Here's how the part is built. I have some questions about the finished solid (model axes, mm). Face numbers are marked on the shaded views. A direction names the side the tool comes from. Give positions to 0.01 mm unless a question says otherwise; leave off trailing zeros. Write each loop counter-clockwise with the first axis right and the second up, starting at its lowest first coordinate (ties: lowest second). Pieces come first, ordered by that corner, then holes. Notation, with made-up numbers: (-35, 73.5) - (-27, 73.5) arc R25 ccw to (-27, 96.5) - close; hole circle Ø11 at (50, -6). An arc over 180 degrees is marked (long way). Use a Markdown table: item, result.
Autodesk Inventor part; units mm, degrees
ref_plane "YZ Plane" through (0, 0, 0) normal (1, 0, 0) x (0, 1, 0)
ref_plane "XZ Plane" through (0, 0, 0) normal (0, 1, 0) x (-1, 0, 0)
ref_plane "XY Plane" through (0, 0, 0) normal (0, 0, 1) x (1, 0, 0)
sketch "Sketch1" plane through (0, 0, 0) normal (0, 1, 0) x (-1, 0, 0)
  line L0 (-11.9316, 12.465) -> (11.9317, 12.465)
  line L1 (11.9317, 12.465) -> (11.9316, -12.465)
  line L2 (11.9316, -12.465) -> (-11.9317, -12.465)
  line L3 (-11.9317, -12.465) -> (-11.9316, 12.465)
  line L4 (-11.9316, 12.465) -> (11.9316, -12.465) construction
  line L5 (11.9317, 12.465) -> (-11.9317, -12.465) construction
  circle A0 centre (10.0076, 9.4933) radius 1.0351
  line L6 (0, 0) -> (10.0076, 0) construction
  line L7 (10.0076, 0) -> (10.0076, 9.4933) construction
  line L8 (4.7752, 0) -> (4.7752, 3.1605) construction
  circle A1 centre (10.0076, -9.4933) radius 1.0351
  circle A2 centre (-0.4572, 9.4933) radius 1.0351
  circle A3 centre (-0.4572, -9.4933) radius 1.0351
  dimension "d0" = 24.9301
  dimension "d1" = 23.8633
  dimension "d2" = 2.0701
  dimension "d3" = 1.9241
  dimension "d5" = 5.2324
  dimension "d16" = 18.9865
extrude "Extrusion1" add sketch "Sketch1" along normal blind 1.016
sketch "Sketch2" plane through (0, 1.016, 0) normal (0, 1, 0) x (1, 0, 0)
  line L0 (4.2101, -4.21) -> (-4.21, -4.21)
  line L1 (-4.21, -4.21) -> (-4.21, 4.21)
  line L2 (-4.21, 4.21) -> (4.2101, 4.2101)
  line L3 (4.2101, 4.2101) -> (4.2101, -4.21)
  line L4 (4.2101, -4.21) -> (-4.21, 4.21) construction
  line L5 (-4.21, -4.21) -> (4.2101, 4.2101) construction
  point P0 (0, 0)
  dimension "d8" = 8.4201
  dimension "d9" = 8.4201
extrude "Extrusion2" add sketch "Sketch2" along normal blind 3.81
sketch "Sketch3" plane through (0, 0, 0) normal (0, -1, 0) x (1, 0, 0)
  line L0 (11.9316, 12.465) -> (11.9317, -12.465)
  line L1 (6.5977, 9.7536) -> (11.9317, 9.7536)
  line L2 (11.9317, 9.7536) -> (11.9317, -9.7536)
  line L3 (11.9317, -9.7536) -> (6.5977, -9.7536)
  line L4 (6.5977, -9.7536) -> (6.5977, 9.7536)
  line L5 (6.5977, 9.7536) -> (11.9317, -9.7536) construction
  line L6 (11.9317, 9.7536) -> (6.5977, -9.7536) construction
  line L7 (0, 0) -> (9.2647, 0) construction
  dimension "d12" = 5.334
  dimension "d13" = 19.5072
extrude "Extrusion3" add sketch "Sketch3" along normal blind 2.1844
properties part number "Camera"
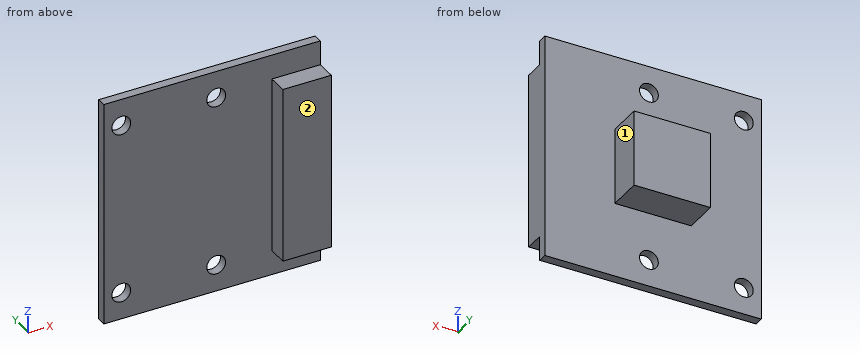
Item 1: Will these pins go through, and if not, where does the flat tip stop? pin 1 Ø1.1 at (x, y) = (9.5, -1) entering from +Z; pin 2 Ø1.9 at (y, z) = (4, -1.5) entering from -X; pin 3 Ø1.9 at (x, y) = (-2, 4) entering from -Z; pin 4 Ø1.2 at (x, z) = (0.46, 9.49) entering from -Y.
Values:
| item | result |
|---|---|
| pin 1 | stops at z = 9.75 |
| pin 2 | stops at x = -4.21 |
| pin 3 | stops at z = -4.21 |
| pin 4 | passes through |
Item 2: If we section it at C-C, the plane z = 6.5: Write out the boundary of the cut face in (x, y), plus the area to 3 significant figures.
Values:
| item | result |
|---|---|
| outline | (-11.93, 0) - (6.6, 0) - (6.6, -2.18) - (11.93, -2.18) - (11.93, 1.02) - (-11.93, 1.02) - close |
| area | 35.9 mm2 |
Item 3: For the marked faces 1 and 2, which set-ups out of +Z, -Z, +X, -X, +Y, -Y let a thin tool reach every point of the face, with its end or its side?
Values:
| item | result |
|---|---|
| face 1 | +Z, -Z, +X, +Y |
| face 2 | +Z, -Z, +X, -X, -Y |
Item 4: If we section it at D-D, the plane y = 4: Write out the boundary of the cut face in (x, z).
Values:
| item | result |
|---|---|
| outline | (-4.21, -4.21) - (4.21, -4.21) - (4.21, 4.21) - (-4.21, 4.21) - close |
Item 5: I need wall thicknesses on line 1 along Z through (x, y) = (-10, 0.25) (3 decimals); line 2 along Y through (x, z) = (-9.75, 3.5); line 3 along X through (y, z) = (-1.25, 7.25). Which ranges of each line are inside material? Lowest first, please. Write a range as [from, to].
Values:
| item | result |
|---|---|
| line 1 | z = [-12.465, -10.528], [-8.458, 8.458], [10.528, 12.465] |
| line 2 | y = [0, 1.02] |
| line 3 | x = [6.6, 11.93] |
Item 6: If we section it at A-A, the plane y = 0.5: Write out the boundary of the cut face in (x, z) (3 decimals), plus the area to 3 significant figures.
Values:
| item | result |
|---|---|
| outline | (-11.932, -12.465) - (11.932, -12.465) - (11.932, 12.465) - (-11.932, 12.465) - close; hole circle Ø2.07 at (-10.008, -9.493); hole circle Ø2.07 at (-10.008, 9.493); hole circle Ø2.07 at (0.457, -9.493); hole circle Ø2.07 at (0.457, 9.493) |
| area | 581 mm2 |
Item 7: If we section it at B-B, the plane x = -1.5: Write out the boundary of the cut face in (y, z) (3 decimals), plus the area to 3 significant figures.
Values:
| item | result |
|---|---|
| outline | (0, -12.465) - (1.016, -12.465) - (1.016, -4.21) - (4.826, -4.21) - (4.826, 4.21) - (1.016, 4.21) - (1.016, 12.465) - (0, 12.465) - close |
| area | 57.4 mm2 |
